Part model, mm, in its own coordinate system. A direction names the side the tool comes from. Round coordinates to 2 decimals unless told otherwise and drop trailing zeros. Write each loop counter-clockwise with the first axis right and the second up, starting at its lowest first coordinate (ties: lowest second). Pieces come first, ordered by that corner, then holes. Notation, with made-up numbers: (26, 79.5) -> (74, 79.5) arc R25 ccw to (74, 99.5) -> close; hole circle Ø3 at (15, 77). An arc over 180 degrees is marked (long way). Use CSV: the item, a comma, the result in double quotes. Start each with the question number.
(1) Saw through at C-C (x = -241.5). Give the cut face in (y, z), plus the area to 3 significant figures.
(2) Saw through at B-B (y = -41.5). Give the cut face in (x, z).
(3) Drop flat-ended pins along their axis: pin 1 (2 mm diameter, centred on y = 25, z = -127.5, fed in from -X); pin 2 (4 mm diameter, centred on x = 5, z = -45.5, fed in from +Y); pin 3 (1.5 mm diameter, centred on y = 11, z = -178.5, fed in from -X). Give the stop position or say it passes through.
(4) Probe line 1 (X direction, y = -26, z = -16.5); line 2 (X direction, y = -46, z = -71.5); line 3 (X direction, y = 27, z = -154.5). List the from-to ranges inside material, lowest first. Write a range as [from, to].
(5) Saw through at D-D (y = 55). Give the cut face in (x, z), plus the area to 3 significant figures.
(6) Which spindle directions (+Z, -Z, +X, -X, +Y, -Y) get a long thin tool onto all of the face, cutting with end or side? Do faces 1 (the cylindrical face through (-1.26, -17.39, -98.6)), 2 (the flat face through (7, 25.119, -99)). Say none if no direction does.
(7) Saw through at A-A (z = -60.5). Give the cut face in (x, y), plus the area to 3 significant figures.
```python
from build123d import *

# Parameters (mm, degrees)
BOSS_EXTRUDE1_DEPTH   = 200
BODY_MOVE_COPY1_ANGLE = 180


with BuildPart() as part:
    # Sketch2 → Boss-Extrude1 (new body)
    with BuildSketch(Plane.XY):
        with BuildLine():
            Line((332.081911263, 10.118919234), (232.081911263, 65.118919234))
            Line((232.081911263, 65.118919234), (72.081911263, 65.118919234))
            Line((72.081911263, 65.118919234), (42.081911263, 25.118919234))
            Line((42.081911263, 25.118919234), (-57.918088737, 25.118919234))
            ThreePointArc((-57.918088737, 25.118919234), (-64.989156549, 22.189987046), (-67.918088737, 15.118919234))
            Line((-67.918088737, 15.118919234), (-67.918088737, -54.881080766))
            Line((-67.918088737, -54.881080766), (-35.418088737, -54.881080766))
            ThreePointArc((-35.418088737, -54.881080766), (2.081911263, -17.381080766), (39.581911263, -54.881080766))
            Line((39.581911263, -54.881080766), (219.581911263, -54.881080766))
            ThreePointArc((219.581911263, -54.881080766), (257.081911263, -17.381080766), (294.581911263, -54.881080766))
            Line((294.581911263, -54.881080766), (332.081911263, -54.881080766))
            Line((332.081911263, -54.881080766), (332.081911263, 10.118919234))
        make_face()
    extrude(amount=BOSS_EXTRUDE1_DEPTH)


with BuildPart() as part_1:
    # Body-Move/Copy1: moved
    add(part.part.rotate(Axis((0, 0, 0), (0, 1, 0)), BODY_MOVE_COPY1_ANGLE))


solid = part_1.part
```
Answers:
1,outline,"(-20.77, -200) -> (59.94, -200) -> (59.94, 0) -> (-20.77, 0) -> close"
1,area,"16,100 mm²"
2,outline,"(-332.08, -200) -> (-292.11, -200) -> (-292.11, 0) -> (-332.08, 0) -> close; (-222.05, -200) -> (-37.11, -200) -> (-37.11, 0) -> (-222.05, 0) -> close; (32.95, -200) -> (67.92, -200) -> (67.92, 0) -> (32.95, 0) -> close"
3,pin 1,"stops at x = -306.84"
3,pin 2,"stops at y = 25.12"
3,pin 3,"stops at x = -331.84"
4,line 1,"x = [-332.08, -281], [-233.16, -26], [21.84, 67.92]"
4,line 2,"x = [-332.08, -293.52], [-220.65, -38.52], [34.35, 67.92]"
4,line 3,"x = [-301.39, -43.49]"
5,outline,"(-250.48, -200) -> (-64.49, -200) -> (-64.49, 0) -> (-250.48, 0) -> close"
5,area,"37,200 mm²"
6,face 1,"+Z, -Z, -Y"
6,face 2,"+Z, -Z, +X, +Y"
7,outline,"(-332.08, -54.88) -> (-294.58, -54.88) arc R37.5 cw to (-219.58, -54.88) -> (-39.58, -54.88) arc R37.5 cw to (35.42, -54.88) -> (67.92, -54.88) -> (67.92, 15.12) arc R10 ccw to (57.92, 25.12) -> (-42.08, 25.12) -> (-72.08, 65.12) -> (-232.08, 65.12) -> (-332.08, 10.12) -> close"
7,area,"35,800 mm²"
